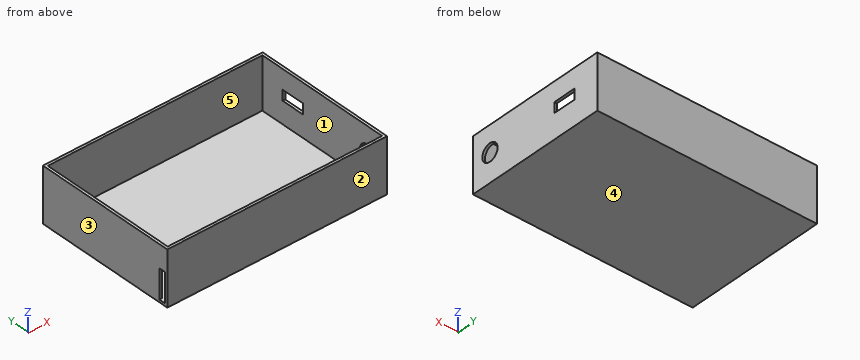
```python
from build123d import *

# Parameters (mm, degrees)
SKETCH1_W           = 170
SKETCH1_H           = 110
BOSS_EXTRUDE1_DEPTH = 2
SKETCH2_W           = 170
SKETCH2_H           = 110
SKETCH2_W_2         = 166
SKETCH2_H_2         = 106
BOSS_EXTRUDE2_DEPTH = 40
SKETCH3_R           = 6.75
SKETCH3_W           = 8
SKETCH3_H           = 18
CUT_EXTRUDE1_DEPTH  = 2
SKETCH4_W           = 22.608078914
SKETCH4_H           = 5
CUT_EXTRUDE2_DEPTH  = 2


with BuildPart() as part:
    # Sketch1 → Boss-Extrude1 (new body)
    with BuildSketch(Plane.XY):
        Rectangle(SKETCH1_W, SKETCH1_H)
    extrude(amount=BOSS_EXTRUDE1_DEPTH)

    # Sketch2 → Boss-Extrude2 (add)
    with BuildSketch(Plane.XY.offset(2)):
        Rectangle(SKETCH2_W, SKETCH2_H)
        Rectangle(SKETCH2_W_2, SKETCH2_H_2, mode=Mode.SUBTRACT)
    extrude(amount=BOSS_EXTRUDE2_DEPTH)

    # Sketch3 → Cut-Extrude1 (cut)
    with BuildSketch(Plane(origin=(85, 0, 0), x_dir=(0, 0, -1), z_dir=(1, 0, 0))):
        with Locations(Location((-22, -39.991227395, 0), (0, 0, 90))):
            Circle(SKETCH3_R)
        with Locations((-23, 26)):
            Rectangle(SKETCH3_W, SKETCH3_H)
    extrude(amount=-CUT_EXTRUDE1_DEPTH, mode=Mode.SUBTRACT)

    # Sketch4 → Cut-Extrude2 (cut)
    with BuildSketch(Plane.ZY.offset(85)):
        with Locations((13.304039457, -50.5)):
            Rectangle(SKETCH4_W, SKETCH4_H)
    extrude(amount=-CUT_EXTRUDE2_DEPTH, mode=Mode.SUBTRACT)


solid = part.part
```
Check sheet for the modelled part. Datum: model origin and axes. Units: mm. Face numbers are marked on the shaded views. A direction names the side the tool comes from. Give positions to 0.01 mm unless a question says otherwise; leave off trailing zeros. Loops run counter-clockwise (first coordinate to the right, second up) from the corner with the lowest first, then second, coordinate; pieces in that order, holes last. Notation, with made-up numbers: M 69,-12.5 L 113,-12.5 A13 cw 113,-5.5 Z; hole C 23.5,7.5 d1. An arc over 180 degrees is marked long. Answer in a Markdown table with one row per item.
1) Cross-section at B-B (z = 22). Enter the section's corners in (x, y).
Solutions:
| item | result |
|---|---|
| outline | M -85,-55 L 85,-55 L 85,-46.74 L 83,-46.74 L 83,-53 L -85,-53 Z; M -85,-48 L -83,-48 L -83,53 L 83,53 L 83,35 L 85,35 L 85,55 L -85,55 Z; M 83,-33.24 L 85,-33.24 L 85,17 L 83,17 Z |
2) Thickness scan on line 1 (X direction, y = 13, z = 17); line 2 (Y direction, x = 18, z = 10); line 3 (Z direction, x = 28, y = -45). Record the ranges inside material, lowest first.
Solutions:
| item | result |
|---|---|
| line 1 | x = -85 to -83, 83 to 85 |
| line 2 | y = -55 to -53, 53 to 55 |
| line 3 | z = 0 to 2 |
3) Cross-section at C-C (x = -46). Enter the section's corners in (y, z), plus the area to 3 significant figures.
Solutions:
| item | result |
|---|---|
| outline | M -55,0 L 55,0 L 55,42 L 53,42 L 53,2 L -53,2 L -53,42 L -55,42 Z |
| area | 380 mm^2 |
4) Cross-section at A-A (z = 35). Enter the section's corners in (x, y), plus the area to 3 significant figures.
Solutions:
| item | result |
|---|---|
| outline | M -85,-55 L 85,-55 L 85,55 L -85,55 Z; hole M -83,-53 L 83,-53 L 83,53 L -83,53 Z |
| area | 1,100 mm^2 |
5) Mould release check, pull along X, two halves, no side actions. Record for the marked faces 1, 2 and 3: released by +X, released by -X, zero draft, split by the parting line, or undercut.
Solutions:
| item | result |
|---|---|
| face 1 | undercut |
| face 2 | zero draft |
| face 3 | released by -X |
6) Depth check by flat-ended pin: pin 1 (6 mm diameter, centred on x = 23.5, y = 38.5, fed in from +Z). Enter the tip coordinate at first touch or a pass-through.
Solutions:
| item | result |
|---|---|
| pin 1 | stops at z = 2 |
7) Cross-section at D-D (y = 41). Enter the section's corners in (x, z), plus the area to 3 significant figures.
Solutions:
| item | result |
|---|---|
| outline | M -85,0 L 85,0 L 85,42 L 83,42 L 83,2 L -83,2 L -83,42 L -85,42 Z |
| area | 500 mm^2 |
8) Tool access check on the marked faces 4 and 5. Record the directions out of +Z, -Z, +X, -X, +Y, -Y that give a thin tool (end or side, any length) a straight path to the whole face; none if there is none.
Solutions:
| item | result |
|---|---|
| face 4 | -Z, +X, -X, +Y, -Y |
| face 5 | +Z |
